Geometry check sheet. Reference: drawing and pictorial views, mm from the part's lowest x, y, z. A direction names the side the tool comes from. Give positions to 0.01 mm unless a question says otherwise; leave off trailing zeros. Write each loop counter-clockwise with the first axis right and the second up, starting at its lowest first coordinate (ties: lowest second). Pieces come first, ordered by that corner, then holes. Notation, with made-up numbers: M 63.25,65.25 L 82.25,65.25 A25 cw 82.25,84.25 Z; hole C 56,7 d6. An arc over 180 degrees is marked long. Write item = value, one per line. Start each with the question number.
1) Mould release check, pull along Z, two halves, no side actions. Record for the marked faces 1, 2, 3 and 4: released by +Z, released by -Z, zero draft, split by the parting line, or undercut.
2) Cross-section at B-B, the plane z = 7.1. Record the cut outline in (x, y).
3) Go/stop test with flat-tipped pins: pin 1 (3 mm diameter, centred on x = 1.5, z = 3.5, fed in from +Y); pin 2 (0.6 mm diameter, centred on x = 7, y = 3.5, fed in from -Z); pin 3 (4 mm diameter, centred on x = 7, y = 9.5, fed in from +Z). Record where each tip stops, or that it passes through.
4) Cross-section at D-D, the plane x = 8.25. Record the cut outline in (y, z).
5) Scan lines: line 1 along Y through (x, z) = (0.9, 7.1); line 2 along X through (y, z) = (12.5, 10.5); line 3 along Z through (x, y) = (1.25, 7.75). Record each from-to range of solid material in increasing order. Write a range as [from, to].
6) Cross-section at A-A, the plane x = 2.25. Record the cut outline in (y, z).
7) Access from +Z, -Z, +X, -X, +Y, -Y to the whole of each face (thin tool, end or side, straight path). Record for the marked faces 5, 6 and 7.
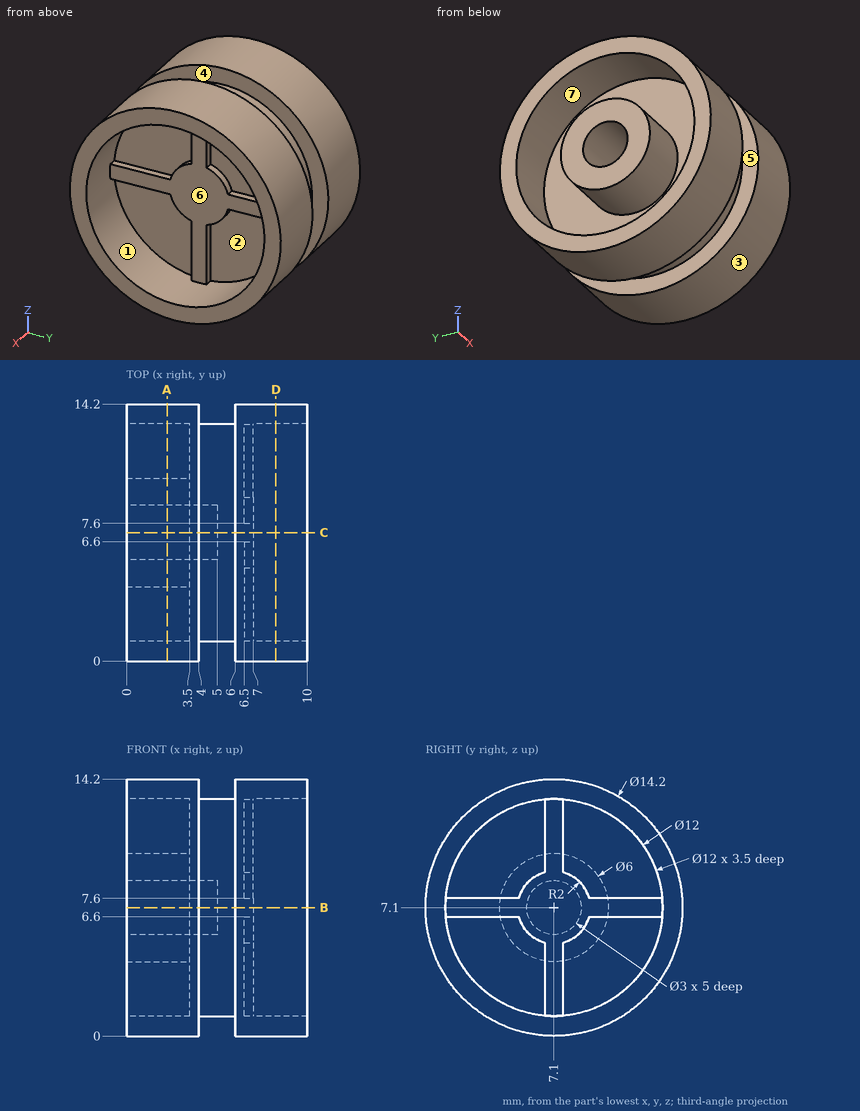
Reply:
q1.face_1 = undercut
q1.face_2 = undercut
q1.face_3 = split by the parting line
q1.face_4 = zero draft
q2.outline = M 0,0 L 4,0 L 4,1.1 L 6,1.1 L 6,0 L 10,0 L 10,1.1 L 7,1.1 L 7,13.1 L 10,13.1 L 10,14.2 L 6,14.2 L 6,13.1 L 4,13.1 L 4,14.2 L 0,14.2 L 0,13.1 L 3.5,13.1 L 3.5,10.1 L 0,10.1 L 0,8.6 L 5,8.6 L 5,5.6 L 0,5.6 L 0,4.1 L 3.5,4.1 L 3.5,1.1 L 0,1.1 Z
q3.pin_1 = 13.88
q3.pin_2 = 0.81
q3.pin_3 = 14.19
q4.outline = C 7.1,7.1 d14.2; hole C 7.1,7.1 d12
q5.line_1 = [0, 1.1], [4.1, 5.6], [8.6, 10.1], [13.1, 14.2]
q5.line_2 = [0, 4], [6, 10]
q5.line_3 = [0.03, 1.14], [4.17, 5.75], [8.45, 10.03], [13.06, 14.17]
q6.outline = C 7.1,7.1 d14.2; C 7.1,7.1 d6; hole C 7.1,7.1 d12; hole C 7.1,7.1 d3
q7.face_5 = none
q7.face_6 = +X
q7.face_7 = -X
